Part model, mm, in its own coordinate system. A direction names the side the tool comes from. Round coordinates to 2 decimals unless told otherwise and drop trailing zeros. Loops run counter-clockwise (first coordinate to the right, second up) from the corner with the lowest first, then second, coordinate; pieces in that order, holes last. Notation, with made-up numbers: M 5.25,81 L 15.25,81 A22 cw 15.25,90 Z; hole C -23.5,27.25 d5. An arc over 180 degrees is marked long. Answer as CSV lines item,"result". Start each with the question number.
Item 1: Band-saw the part on C-C (x = -1). Give the cut face in (y, z), and give its area (3 significant figures).
Item 2: Which spindle directions (+Z, -Z, +X, -X, +Y, -Y) get a long thin tool onto all of the face, cutting with end or side? Do faces 1 (the flat face through (11, -1, -12)), 2 (the flat face through (1.6, -1, 6)), 3 (the flat face through (-10, -1, -15)). Say none if no direction does.
Item 3: Band-saw the part on B-B (y = -1.7). Give the cut face in (x, z).
Item 4: Drop flat-ended pins along their axis: pin 1 Ø0.9 at (x, y) = (0.5, -1.5) entering from +Z; pin 2 Ø0.6 at (x, y) = (-10.5, -1.5) entering from -Z; pin 3 Ø0.9 at (y, z) = (-1.5, -14.5) entering from +X. Give the stop position or say it passes through.
Item 5: Mould opens along X. For faces 4 (the flat face through (-12, -1, 0)), 5 (the flat face through (-7, -1, 12)), 6 (the flat face through (-1.6, -1, 6)) say: pulls with the +X half, pulls with the -X half, needs draft (parallel to the pull), parting line crosses it, or undercut.
Item 6: Wall check: line 1 (X direction, y = -0.7, z = 1.5); line 2 (Z direction, x = -0.5, y = -1.7); line 3 (Z direction, x = 10.25, y = -2.4). Give the ranges that are in metal, low to high.
Item 7: Band-saw the part on A-A (z = 1.75). Give the cut face in (x, y).
```python
from build123d import *

# Parameters (mm, degrees)
F0_W     = 20
F0_H     = 5
F1_DEPTH = 3


with BuildPart() as f1:
    # F0 (on Front) → F1 (new body)
    with BuildSketch(Plane.XZ):
        Polygon((-12, 12), (-12, -12), (-10, -12), (10, -12), (12, -12), (12, 12), (1.6, 12), (1.6, 0), (-1.6, 0), (-1.6, 12), align=None)
        with Locations((0, -14.5)):
            Rectangle(F0_W, F0_H)
    extrude(amount=F1_DEPTH)


solid = f1.part
```
Answer block:
1,outline,"M -3,-17 L 0,-17 L 0,0 L -3,0 Z"
1,area,"51.0 mm^2"
2,face 1,"-Z, +X, +Y, -Y"
2,face 2,"+Z, +Y, -Y"
2,face 3,"-Z, -X, +Y, -Y"
3,outline,"M -12,-12 L -10,-12 L -10,-17 L 10,-17 L 10,-12 L 12,-12 L 12,12 L 1.6,12 L 1.6,0 L -1.6,0 L -1.6,12 L -12,12 Z"
4,pin 1,"stops at z = 0"
4,pin 2,"stops at z = -12"
4,pin 3,"stops at x = 10"
5,face 4,"pulls with the -X half"
5,face 5,"needs draft"
5,face 6,"undercut"
6,line 1,"x = -12 to -1.6, 1.6 to 12"
6,line 2,"z = -17 to 0"
6,line 3,"z = -12 to 12"
7,outline,"M -12,-3 L -1.6,-3 L -1.6,0 L -12,0 Z; M 1.6,-3 L 12,-3 L 12,0 L 1.6,0 Z"
